The listing builds one solid part. Answer for the finished solid, in the listing's coordinates (mm). Coordinates: 2 decimals unless noted, no trailing zeros. Order: outer loops, then holes, each group sorted by start corner. A loop starts at its lowest first (then second) coordinate and runs counter-clockwise, first axis right, second up. Notation, with made-up numbers: (59.25, -22.5) -> (118.25, -22.5) arc R16 cw to (118.25, -9.5) -> close; hole circle Ø2 at (-12, 86.25). An arc over 180 degrees is marked (long way). Return JSON: item names as keys, results as strings.
from build123d import *

# Parameters (mm, degrees)
FILLET1_R    = 0.1
SKETCH3_W    = 0.74
SKETCH3_H    = 2.8
SKETCH4_W    = 0.74
SKETCH4_H    = 1.054964664
RECPAT_COUNT = 2
RECPAT_ANGLE = 90


with BuildPart() as part:
    # BodySke → Base-Revolve (revolve)
    with BuildSketch(Plane.XY):
        with BuildLine():
            Line((2.4, 1.5), (2.4, 2.8))
            Line((2.4, 2.8), (1.003501533, 2.8))
            ThreePointArc((1.003501533, 2.8), (0.873295971, 2.76653015), (0.775371599, 2.674418605))
            ThreePointArc((0.775371599, 2.674418605), (0.197753546, 1.392274756), (0, 0))
            Line((0, 0), (18.4, 0))
            Line((18.4, 0), (18.4, 1.5))
            Line((18.4, 1.5), (2.4, 1.5))
        make_face()
    revolve(axis=Axis((-25.4, 0, 0), (1, 0, 0)))

    # Fillet1
    fillet1_edges = [part.edges().sort_by_distance(p)[0] for p in [
        (2.4, -1.5, 0),
    ]]
    fillet(fillet1_edges, radius=FILLET1_R)

    # Sketch3 → Recess section 0
    with BuildSketch(Plane(origin=(0, 0, 0), x_dir=(0, 0, -1), z_dir=(1, 0, 0))):
        Rectangle(SKETCH3_W, SKETCH3_H)
    # Sketch4 → Recess section 1
    with BuildSketch(Plane(origin=(1.75, 0, 0), x_dir=(0, 0, -1), z_dir=(1, 0, 0))):
        Rectangle(SKETCH4_W, SKETCH4_H)
    recess = loft(mode=Mode.SUBTRACT)

    # RecPat: Recess ×2 about axis
    recpat_axis = Axis((0, 0, 0), (1, 0, 0))
    for i in range(1, RECPAT_COUNT):
        add(recess.rotate(recpat_axis, i * RECPAT_ANGLE / (RECPAT_COUNT - 1)), mode=Mode.SUBTRACT)

    # RecCorSke → RecessCore (revolve, cut)
    with BuildSketch(Plane.XY):
        Polygon((0, 0), (0, 0.678371921), (1.75, 0.556), (1.930655351, 0), align=None)
    revolve(axis=Axis((-3.175, 0, 0), (1, 0, 0)), mode=Mode.SUBTRACT)


solid = part.part
1. Determine the mould class of faces 1 (the face through (18.4, 0, 0)), 2 (the face through (1.7, -2.8, 0.1)), 3 (the face through (1.92, 0.03, 0.01)) for opening direction Z: pulls with the +Z half, pulls with the -Z half, needs draft (parallel to the pull), parting line crosses it, or undercut.
Answer block:
{"face 1": "needs draft", "face 2": "parting line crosses it", "face 3": "undercut"}
2. The part is cut by section A-A on x = 16. Give the vertices of the cut face in (y, z), and give its area (3 significant figures).
Answer block:
{"outline": "circle Ø3 at (0, 0)", "area": "7.07 mm2"}
3. Each of these flat-tipped pins is pushed along its axis until it touches: pin 1 Ø1.5 at (x, z) = (5.5, -0.5) entering from -Y; pin 2 Ø1 at (x, y) = (7.5, 1.5) entering from -Z; pin 3 Ø2 at (y, z) = (0, -1) entering from -X. Where does it stop, or does it pass through?
Answer block:
{"pin 1": "stops at y = -1.5", "pin 2": "stops at z = -1.12", "pin 3": "stops at x = 0.05"}
4. Consider line 1 (X direction, y = 1.55, z = 1.7); line 2 (Z direction, x = 4, y = 0.05); line 3 (Y direction, x = 16.75, z = -0.7). Determine where each line is inside the solid, lowest interval first. Write a range as from..to.
Answer block:
{"line 1": "x = 0.56..2.4", "line 2": "z = -1.5..1.5", "line 3": "y = -1.33..1.33"}
